CAD build for the part. Positions are in the model's coordinates, mm. A direction names the side the tool comes from. Round coordinates to 2 decimals unless told otherwise and drop trailing zeros. Loops run counter-clockwise (first coordinate to the right, second up) from the corner with the lowest first, then second, coordinate; pieces in that order, holes last. Notation, with made-up numbers: M 61.25,-38 L 82.25,-38 A33 ccw 82.25,-3 Z; hole C -38.75,29.5 d10. An arc over 180 degrees is marked long. Use a Markdown table: item, result. Add a question column.
(1) Band-saw the part on B-B, the plane x = 18. Write the cut outline in (y, z), and give its area (3 significant figures).
(2) Wall check: L1, parallel to Y at x = 9, z = 4.25; L2, parallel to X at y = 134.5, z = 2.3; L3, parallel to Z at x = -5, y = 27. Give the ranges that are in metal, low to high.
(3) Flat gauge pins, fed straight in: P1, Ø0.9, axis at y = 64.5, z = 3, coming from the -X side; P2, Ø1.5, axis at x = -29.5, y = 34.5, coming from the +Z side; P3, Ø1.5, axis at x = 51.5, z = 3, coming from the +Y side. Where does each tip first touch, or does it go through?
(4) Two-plate mould, pull along X, no slides. Class faces 1 (the face through (19, 8, 2)), 2 (the face through (24, 78, 2)), 3 (the face through (-40.34, 142.22, 3.52)), 4 (the face through (90.43, 11.45, 3.52)): released by +X, released by -X, zero draft, split by the parting line, or undercut.
(5) Band-saw the part on C-C, the plane y = 42. Write the cut outline in (x, z).
(6) Band-saw the part on A-A, the plane z = 3.35. Write the cut outline in (x, y).
(7) Which spindle directions (+Z, -Z, +X, -X, +Y, -Y) get a long thin tool onto all of the face, cutting with end or side? Do faces 5 (the face through (90.51, 142.22, 3.52)), 6 (the face through (24, 78, 0)), 7 (the face through (-40.34, 11.53, 3.52)). Say none if no direction does.
from build123d import *

# Parameters (mm, degrees)
F0_W     = 144
F0_H     = 144
F2_DEPTH = 2
F1_W     = 133.7
F1_H     = 133.7
F1_W_2   = 129.7
F1_H_2   = 129.7
F3_DEPTH = 5
F4_R     = 5


with BuildPart() as f2:
    # F0 (on Top) → F2 (new body)
    with BuildSketch(Plane.XY):
        with Locations((25.086074, 76.876128)):
            Rectangle(F0_W, F0_H)
    extrude(amount=F2_DEPTH)

    # F1 (on face) → F3 (join)
    with BuildSketch(Plane.XY):
        with Locations((25.086074, 76.876128)):
            Rectangle(F1_W, F1_H)
        with Locations((25.086074, 76.876128)):
            Rectangle(F1_W_2, F1_H_2, mode=Mode.SUBTRACT)
    extrude(amount=F3_DEPTH)

    # F4
    f4_edges = [f2.edges().sort_by_distance(p)[0] for p in [
        (-41.763926, 143.726128, 3.5),
        (91.936074, 143.726128, 3.5),
        (-41.763926, 10.026128, 3.5),
        (91.936074, 10.026128, 3.5),
    ]]
    fillet(f4_edges, radius=F4_R)


solid = f2.part
Return value:
| question | item | result |
|---|---|---|
| 1 | outline | M 4.88,0 L 148.88,0 L 148.88,2 L 143.73,2 L 143.73,5 L 141.73,5 L 141.73,2 L 12.03,2 L 12.03,5 L 10.03,5 L 10.03,2 L 4.88,2 Z |
| 1 | area | 300 mm^2 |
| 2 | L1 | 10.03 to 12.03, 141.73 to 143.73 |
| 2 | L2 | -41.76 to -39.76, 89.94 to 91.94 |
| 2 | L3 | 0 to 2 |
| 3 | P1 | x = -41.76 |
| 3 | P2 | z = 2 |
| 3 | P3 | y = 143.73 |
| 4 | face 1 | zero draft |
| 4 | face 2 | undercut |
| 4 | face 3 | released by -X |
| 4 | face 4 | released by +X |
| 5 | outline | M -46.91,0 L 97.09,0 L 97.09,2 L 91.94,2 L 91.94,5 L 89.94,5 L 89.94,2 L -39.76,2 L -39.76,5 L -41.76,5 L -41.76,2 L -46.91,2 Z |
| 6 | outline | M -41.76,15.03 A5 ccw -36.76,10.03 L 86.94,10.03 A5 ccw 91.94,15.03 L 91.94,138.73 A5 ccw 86.94,143.73 L -36.76,143.73 A5 ccw -41.76,138.73 Z; hole M -39.76,12.03 L 89.94,12.03 L 89.94,141.73 L -39.76,141.73 Z |
| 7 | face 5 | +Z, +X, +Y |
| 7 | face 6 | -Z, +X, -X, +Y, -Y |
| 7 | face 7 | +Z, -X, -Y |
